Can you work these out from the model? Positions are in its coordinate system, mm. Coordinates: 2 decimals unless noted, no trailing zeros. Loops run counter-clockwise (first coordinate to the right, second up) from the corner with the lowest first, then second, coordinate; pieces in that order, holes last. Notation, with made-up numbers: M -10,-31 L 25,-31 A19 ccw 25,1 Z; hole C 20.5,1.5 d10. An arc over 180 degrees is marked long. Answer as a JSON object with one key per item and string values. Group by question number.
Item 1: If I drill on line 1 (X direction, y = 3.6, z = 12.7); line 2 (Z direction, x = -38.1, y = 2.1); line 3 (X direction, y = 2.4, z = 12), over which ranges is the centre line in solid material (lowest first)?
Item 2: Suppose I cut it at B-B (x = -12.7). Write out the boundary of the cut face in (y, z), then the cut area to 3 significant figures.
Item 3: We'd pull the mould along Z, two halves only. Please class faces 1 (the flat face through (-50.8, 2, 13)), 2 (the cylindrical face through (-12.971, 2.415, 10.635)), 3 (the cylindrical face through (-0.91, 2.35, 24.45)): +Z half, -Z half, draft (parallel to the pull), parting line (faces both ways), or undercut.
Item 4: Suppose I cut it at C-C (y = 1.8). Write out the boundary of the cut face in (x, z) (3 decimals), then the cut area to 3 significant figures.
Item 5: Suppose I cut it at A-A (z = 12.7). Write out the boundary of the cut face in (x, y), then the cut area to 3 significant figures.
Autodesk Inventor part; units mm, degrees
ref_plane "YZ Plane" through (0, 0, 0) normal (1, 0, 0) x (0, 1, 0)
ref_plane "XZ Plane" through (0, 0, 0) normal (0, 1, 0) x (-1, 0, 0)
ref_plane "XY Plane" through (0, 0, 0) normal (0, 0, 1) x (1, 0, 0)
sketch "Sketch1" plane through (0, 0, 0) normal (0, 1, 0) x (-1, 0, 0)
  line L0 (3.175, 0) -> (47.625, 0)
  line L1 (50.8, 3.175) -> (50.8, 22.225)
  line L2 (47.625, 25.4) -> (3.175, 25.4)
  line L3 (0, 22.225) -> (0, 3.175)
  arc A0 (3.175, 25.4) -> (0, 22.225) centre (3.175, 22.225) ccw
  arc A1 (0, 3.175) -> (3.175, 0) centre (3.175, 3.175) ccw
  arc A2 (47.625, 0) -> (50.8, 3.175) centre (47.625, 3.175) ccw
  arc A3 (50.8, 22.225) -> (47.625, 25.4) centre (47.625, 22.225) ccw
  point P0 (0, 0)
  point P1 (50.8, 25.4)
  point P2 (0, 25.4)
  dimension "d0" = 25.4
  dimension "d1" = 50.8
  dimension "d2" = 3.175
extrude "Extrusion1" add sketch "Sketch1" along normal blind 4.7625
sketch "Sketch2" plane through (0, 4.7625, 0) normal (0, 1, 0) x (1, 0, 0)
  line L0 (-3.175, 0) -> (-47.625, 0)
  line L1 (-50.8, -3.175) -> (-50.8, -22.225)
  line L2 (-47.625, -25.4) -> (-3.175, -25.4)
  circle A0 centre (-38.1, -12.7) radius 2.0828
  circle A1 centre (-12.7, -12.7) radius 2.0828
  point P0 (0, 0)
  dimension "d5" = 4.1656
  dimension "d6" = 12.7
  dimension "d7" = 12.7
  dimension "d10" = 25.4
extrude "Extrusion2" cut sketch "Sketch2" against normal blind 4.7625
properties part number "Spacer" material "Aluminum 6061"
From the geometry:
{
 "1": {"line 1": "-50.8 to -40.18, -36.02 to -14.78, -10.62 to 0", "line 2": "0 to 10.62, 14.78 to 25.4", "line 3": "-50.8 to -40.06, -36.14 to -14.66, -10.74 to 0"},
 "2": {"outline": "M 0,0 L 4.76,0 L 4.76,10.62 L 0,10.62 Z; M 0,14.78 L 4.76,14.78 L 4.76,25.4 L 0,25.4 Z", "area": "101 mm2"},
 "3": {"face 1": "draft", "face 2": "undercut", "face 3": "+Z half"},
 "4": {"outline": "M -50.8,3.175 A3.175 ccw -47.625,0 L -3.175,0 A3.175 ccw 0,3.175 L 0,22.225 A3.175 ccw -3.175,25.4 L -47.625,25.4 A3.175 ccw -50.8,22.225 Z; hole C -38.1,12.7 d4.166; hole C -12.7,12.7 d4.166", "area": "1,250 mm2"},
 "5": {"outline": "M -50.8,0 L -40.18,0 L -40.18,4.76 L -50.8,4.76 Z; M -36.02,0 L -14.78,0 L -14.78,4.76 L -36.02,4.76 Z; M -10.62,0 L 0,0 L 0,4.76 L -10.62,4.76 Z", "area": "202 mm2"}
}
